Part model, mm, in its own coordinate system. Round coordinates to 2 decimals unless told otherwise and drop trailing zeros. Loops run counter-clockwise (first coordinate to the right, second up) from the corner with the lowest first, then second, coordinate; pieces in that order, holes last.
from build123d import *

# Parameters (mm, degrees)
F1_DEPTH = 2
F3_DEPTH = 18
F4_DEPTH = 25
F5_DEPTH = 25
F6_R     = 5


with BuildPart() as f1:
    # F0 (on Front) → F1 (new body)
    with BuildSketch(Plane.XZ):
        Polygon((0, -26.3405761516), (0, 30.6594238484), (-35, 30.6594238484), (-35, -6.3405761516), align=None)
    extrude(amount=F1_DEPTH)

    # F2 (on face) → F3 (join)
    with BuildSketch(Plane.XY.offset(30.6594238484)):
        with BuildLine():
            Line((-3.2919103401, 0), (-1.8350348686, 0))
            ThreePointArc((-1.8350348686, 0), (-2.5634726044, 0.246386627), (-3.2919103401, 0))
        make_face()
        with BuildLine():
            ThreePointArc((-3.1509034742, -2), (-2.5634726044, -2.153613373), (-1.9760417346, -2))
            Line((-1.9760417346, -2), (-3.1509034742, -2))
        make_face()
    extrude(amount=-F3_DEPTH)

    # F2 (on face) → F4 (join)
    with BuildSketch(Plane.XY.offset(30.6594238484)):
        with BuildLine():
            ThreePointArc((-1.9760417346, -2), (-1.5278768715, -1.5598653652), (-1.3634726044, -0.953613373))
            ThreePointArc((-1.3634726044, -0.953613373), (-1.4878041418, -0.4216948092), (-1.8350348686, 0))
            Line((-1.8350348686, 0), (-3.2919103401, 0))
            ThreePointArc((-3.2919103401, 0), (-3.7605012368, -1.0380080009), (-3.1509034742, -2))
            Line((-3.1509034742, -2), (-1.9760417346, -2))
        make_face()
    extrude(amount=F4_DEPTH)

    # F2 (on face) → F5 (join)
    with BuildSketch(Plane.XY.offset(30.6594238484)):
        with BuildLine():
            ThreePointArc((-3.1509034742, -2), (-2.5634726044, -2.153613373), (-1.9760417346, -2))
            Line((-1.9760417346, -2), (-3.1509034742, -2))
        make_face()
        with BuildLine():
            Line((-3.2919103401, 0), (-1.8350348686, 0))
            ThreePointArc((-1.8350348686, 0), (-2.5634726044, 0.246386627), (-3.2919103401, 0))
        make_face()
    extrude(amount=F5_DEPTH)

    # F6
    f6_edges = [f1.edges().sort_by_distance(p)[0] for p in [
        (-35, -1, -6.340576),
    ]]
    fillet(f6_edges, radius=F6_R)


solid = f1.part
1) Mould opens along X. For faces 1 (the face through (-35, -1, 14)), 2 (the face through (0, -1, 2)), 3 (the face through (-18, 0, 9)) say: released by +X, released by -X, zero draft, split by the parting line, or undercut.
Values:
face 1: released by -X
face 2: released by +X
face 3: zero draft
2) Slice it at D-D, the plane x = -21. Give the cut face in (y, z).
Values:
outline: (-2, -14.34) - (0, -14.34) - (0, 30.66) - (-2, 30.66) - close
3) Slice it at C-C, the plane z = 15. Give the cut face in (x, y).
Values:
outline: (-35, -2) - (-3.15, -2) arc R1.2 ccw to (-1.98, -2) - (0, -2) - (0, 0) - (-1.84, 0) arc R1.2 ccw to (-3.29, 0) - (-35, 0) - close
4) Slice it at A-A, the plane z = 46. Give the cut face in (x, y), then the cut area to 3 significant figures.
Values:
outline: circle Ø2.4 at (-2.56, -0.95)
area: 4.52 mm2
5) Slice it at B-B, the plane y = -0.45. Give the cut face in (x, z), then the cut area to 3 significant figures.
Values:
outline: (-35, -3.44) arc R5 ccw to (-32.48, -7.78) - (0, -26.34) - (0, 30.66) - (-1.47, 30.66) - (-1.47, 55.66) - (-3.65, 55.66) - (-3.65, 30.66) - (-35, 30.66) - close
area: 1,700 mm2
6) Drop flat-ended pins along their axis: pin 1 Ø3 at (x, z) = (-21.5, 33) entering from -Y; pin 2 Ø1 at (x, z) = (-23, -13) entering from -Y; pin 3 Ø8 at (x, z) = (-26, 10.5) entering from +Y. Give the stop position or say it passes through.
Values:
pin 1: passes through
pin 2: stops at y = -2
pin 3: stops at y = 0
7) Wall check: line 1 along Y through (x, z) = (-27, 15.5); line 2 along X through (y, z) = (-0.75, 44); line 3 along X through (y, z) = (-0.85, 33). Give the ranges that are in metal, low to high.
Values:
line 1: y = -2 to 0
line 2: x = -3.75 to -1.38
line 3: x = -3.76 to -1.37
